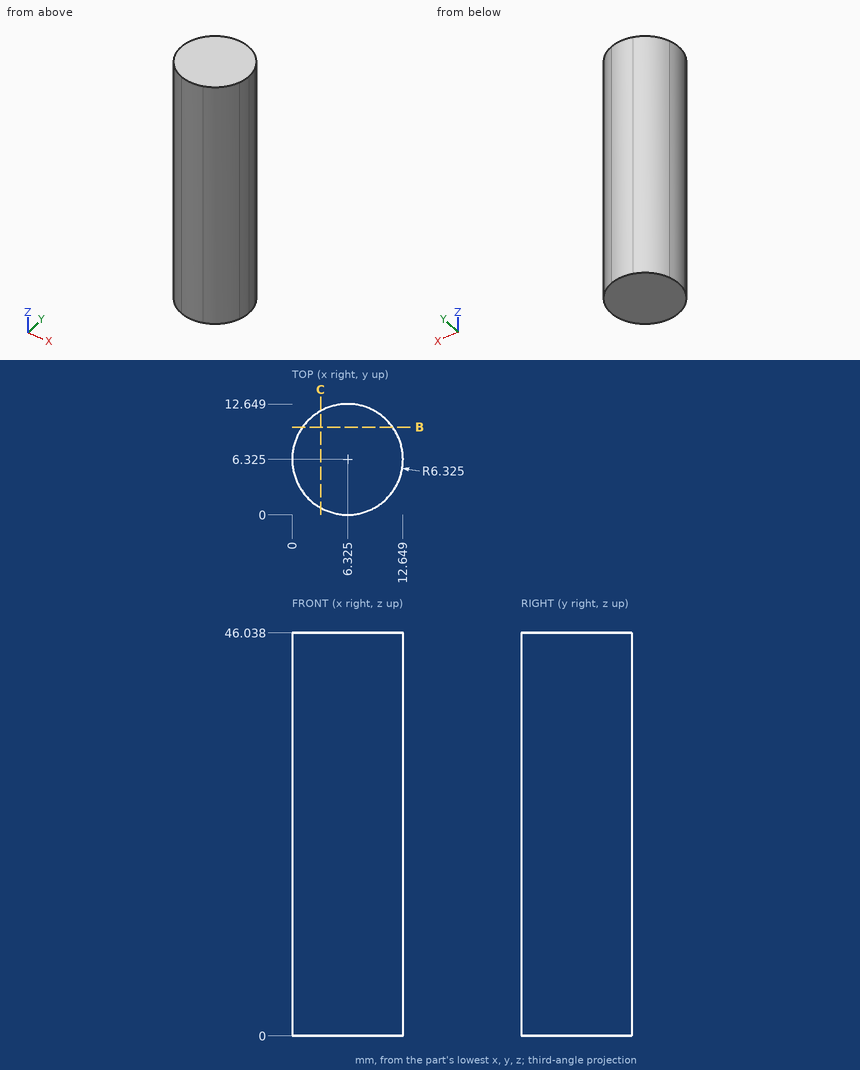
Part print with two shaded views. Sizes in mm from the minimum x, y, z corner. Round coordinates to 2 decimals unless told otherwise and drop trailing zeros. Loops run counter-clockwise (first coordinate to the right, second up) from the corner with the lowest first, then second, coordinate; pieces in that order, holes last. Notation, with made-up numbers: M 45.25,36 L 101.25,36 A27 cw 101.25,67 Z; hole C 66.5,54 d10. An arc over 180 degrees is marked long. Return JSON: item names as keys, results as strings. Group by question number.
(1) Saw through at C-C, the plane x = 3.25. List the corners of the cut face in (y, z).
(2) Wall check: probe 1 along X at (y, z) = (6, 14); probe 2 along Y at (x, z) = (11, 32.5) (1 decimal); probe 3 along X at (y, z) = (9.25, 4). Give the ranges that are in metal, low to high. Write a range as [from, to].
(3) Drop flat-ended pins along their axis: P1, Ø1, axis at y = 8.5, z = 6.5, coming from the +X side; P2, Ø4, axis at y = 4, z = 28.5, coming from the -X side; P3, Ø1.5, axis at y = 1.5, z = 7, coming from the -X side. Give the stop position or say it passes through.
(4) Saw through at B-B, the plane y = 10. List the corners of the cut face in (x, z), and give its area (3 significant figures).
Answer list:
{
 "1": {"outline": "M 0.8,0 L 11.85,0 L 11.85,46.04 L 0.8,46.04 Z"},
 "2": {"probe 1": "[0.01, 12.64]", "probe 2": "[2.1, 10.6]", "probe 3": "[0.72, 11.93]"},
 "3": {"P1": "x = 12.42", "P2": "x = 0.01", "P3": "x = 1.49"},
 "4": {"outline": "M 1.18,0 L 11.47,0 L 11.47,46.04 L 1.18,46.04 Z", "area": "474 mm2"}
}
